from build123d import *

# Parameters (mm, degrees)
F0_R     = 4
F1_DEPTH = 200


with BuildPart() as f1:
    # F0 (on Top) → F1 (new body)
    with BuildSketch(Plane.XY):
        Circle(F0_R)
    extrude(amount=F1_DEPTH)

    # F2 (on Front) → F3 (revolve, cut)
    with BuildSketch(Plane.XZ):
        Polygon((2.5, 2), (2.5, 0), (4, 0), (4, 33.55), (2.5, 32.05), (2.5, 2.7), (2.4, 2.7), (2.4, 2), align=None)
    revolve(axis=Axis((0, 0, 16.025), (0, 0, 1)), mode=Mode.SUBTRACT)

    # F4 (on Front) → F5 (revolve, cut)
    with BuildSketch(Plane.XZ):
        Polygon((0, 200), (0, 61.35), (4, 61.35), (4, 59.35), (3.8, 59.35), (3.8, 58.45), (4, 58.45), (6.54, 58.45), (6.54, 63.53), (4, 63.53), (4, 200), align=None)
    revolve(axis=Axis((0, 0, 130.675), (0, 0, 1)), mode=Mode.SUBTRACT)


solid = f1.part
The model under review builds one solid part; all positions refer to its coordinate system, in mm. A direction names the side the tool comes from. Round coordinates to 2 decimals unless told otherwise and drop trailing zeros. Loops run counter-clockwise (first coordinate to the right, second up) from the corner with the lowest first, then second, coordinate; pieces in that order, holes last. Notation, with made-up numbers: (29.25, 46) -> (47.25, 46) arc R27 cw to (47.25, 78) -> close; hole circle Ø4 at (23.25, 76). An arc over 180 degrees is marked (long way). Answer as CSV lines item,"result".
1) Add section A-A on y = 0. Write out the cut boundary in (x, z), plus the area to 3 significant figures.
Geometry results:
outline,"(-4, 33.55) -> (-2.5, 32.05) -> (-2.5, 2.7) -> (-2.4, 2.7) -> (-2.4, 2) -> (-2.5, 2) -> (-2.5, 0) -> (2.5, 0) -> (2.5, 2) -> (2.4, 2) -> (2.4, 2.7) -> (2.5, 2.7) -> (2.5, 32.05) -> (4, 33.55) -> (4, 58.45) -> (3.8, 58.45) -> (3.8, 59.35) -> (4, 59.35) -> (4, 61.35) -> (-4, 61.35) -> (-4, 59.35) -> (-3.8, 59.35) -> (-3.8, 58.45) -> (-4, 58.45) -> close"
area,"392 mm²"
2) Draft analysis for pull direction Z (two halves, no side actions). For faces 1 (the face through (1.29, 2.024, 2.345)), 2 (the face through (0, 0, 0)), 3 (the face through (-0.867, -3.905, 60.336)), state which applies: pulls with the +Z half, pulls with the -Z half, needs draft (parallel to the pull), parting line crosses it, or undercut.
Geometry results:
face 1,"undercut"
face 2,"pulls with the -Z half"
face 3,"needs draft"
3) To check wall thickness, follow line 1 along X through (y, z) = (0.25, 34.5); line 2 along Z through (x, y) = (-3, 2.5); line 3 along X through (y, z) = (-1.25, 45.5). State the ranges of each line that lie inside material, in increasing order. Write a range as from..to.
Geometry results:
line 1,"x = -3.99..3.99"
line 2,"z = 33.46..58.45, 59.35..61.35"
line 3,"x = -3.8..3.8"
4) For P1, Ø1, axis at x = 3, z = 51, coming from the -Y side; P2, Ø4, axis at y = 0, z = 25, coming from the +X side; P3, Ø1.5, axis at x = -3, z = 36, coming from the -Y side, all flat-tipped, find the tip position at first contact; note any pin that passes through.
Geometry results:
P1,"stops at y = -3.12"
P2,"stops at x = 2.5"
P3,"stops at y = -3.31"
5) Tool access review of faces 4 (the face through (0, 0, 61.35)), 5 (the face through (-3.796, 0.167, 58.894)), 6 (the face through (-0.54, -2.44, 17.17)): name each direction out of +Z, -Z, +X, -X, +Y, -Y from which nothing blocks a thin tool from reaching the whole face with its end or side.
Geometry results:
face 4,"+Z, +X, -X, +Y, -Y"
face 5,"none"
face 6,"-Z"
6) Add section C-C on z = 45. Write out the cut boundary in (x, y), plus the area to 3 significant figures.
Geometry results:
outline,"circle Ø8 at (0, 0)"
area,"50.3 mm²"
7) Add section D-D on z = 28. Write out the cut boundary in (x, y).
Geometry results:
outline,"circle Ø5 at (0, 0)"
